Geometry check sheet. Reference: drawing and pictorial views, mm from the part's lowest x, y, z. A direction names the side the tool comes from. Round coordinates to 2 decimals unless told otherwise and drop trailing zeros. Order: outer loops, then holes, each group sorted by start corner. A loop starts at its lowest first (then second) coordinate and runs counter-clockwise, first axis right, second up.
(1) Sectioned sample at C-C (y = 17.3). Record the boundary of the cut face in (x, z), plus the area to 3 significant figures.
(2) Set-up check for the marked faces 4, 5, 6, 7 and 8: record each of +Z, -Z, +X, -X, +Y, -Y from which the full face is reachable in a straight line by a thin tool's end or side.
(3) Release check for a two-part mould opening along X. For the marked faces 1, 2 and 3 record: +X half, -X half, draft (parallel to the pull), parting line (faces both ways), or undercut.
(4) Material ranges on line 1 along Y through (x, z) = (14, 2.6); line 2 along Z through (x, y) = (27, 17.3); line 3 along Y through (x, z) = (13, 1), recorded low to high.
(5) Sectioned sample at B-B (z = 11.5). Record the boundary of the cut face in (x, y), plus the area to 3 significant figures.
(6) Go/stop test with flat-tipped pins: pin 1 (5 mm diameter, centred on x = 16.5, y = 31.5, fed in from +Z); pin 2 (4.5 mm diameter, centred on x = 32, y = 29.5, fed in from -Z); pin 3 (0.6 mm diameter, centred on x = 28.5, y = 34.5, fed in from +Z); pin 4 (3 mm diameter, centred on x = 14, y = 5.3, fed in from +Z). Record where each tip stops, or that it passes through.
(7) Sectioned sample at D-D (z = 2). Record the boundary of the cut face in (x, y).
(8) Sectioned sample at A-A (x = 31). Record the boundary of the cut face in (y, z), plus the area to 3 significant figures.
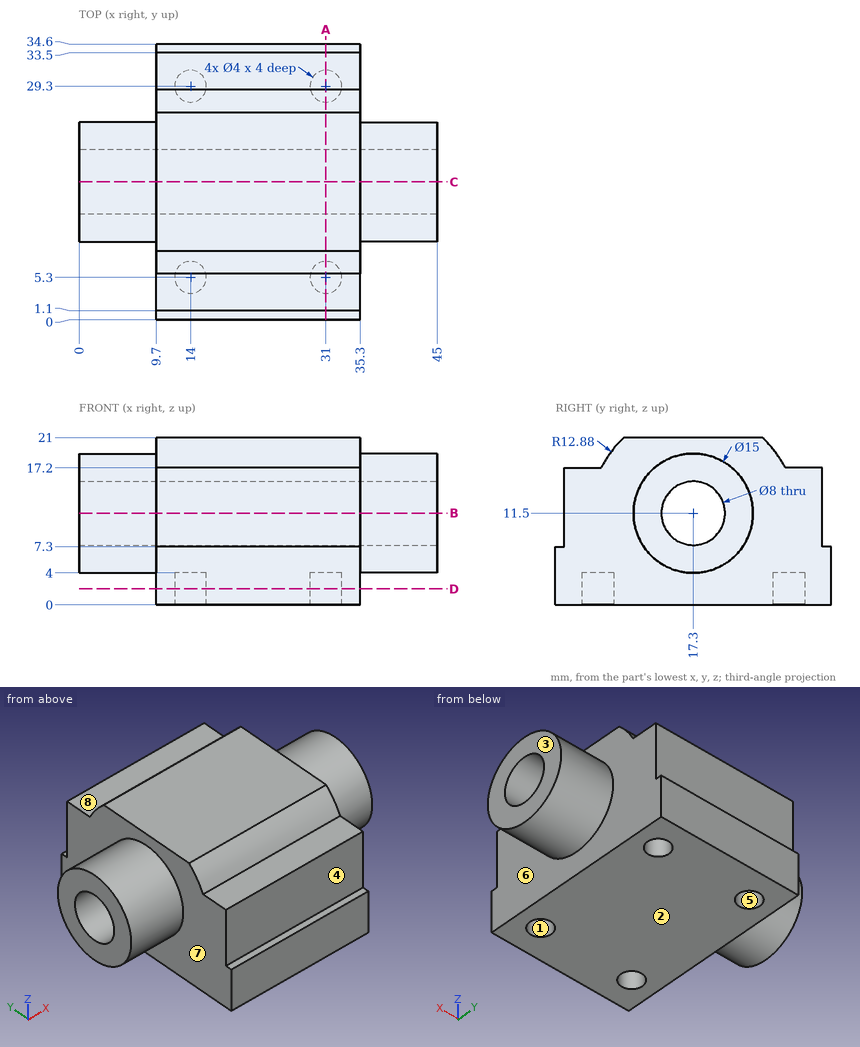
Answer below:
1. outline: (0, 4) - (9.7, 4) - (9.7, 0) - (35.3, 0) - (35.3, 4) - (45, 4) - (45, 7.5) - (0, 7.5) - close; (0, 15.5) - (45, 15.5) - (45, 19) - (35.3, 19) - (35.3, 21) - (9.7, 21) - (9.7, 19) - (0, 19) - close
1. area: 469 mm2
2. face 4: +Z, +X, -X, -Y
2. face 5: -Z
2. face 6: +X
2. face 7: -X
2. face 8: +Z, +X, -X, +Y
3. face 1: undercut
3. face 2: draft
3. face 3: +X half
4. line 1: y = 0 to 3.3, 7.3 to 27.3, 31.3 to 34.6
4. line 2: z = 0 to 7.5, 15.5 to 21
4. line 3: y = 0 to 3.57, 7.03 to 27.57, 31.03 to 34.6
5. outline: (0, 9.8) - (9.7, 9.8) - (9.7, 1.1) - (35.3, 1.1) - (35.3, 9.8) - (45, 9.8) - (45, 13.3) - (0, 13.3) - close; (0, 21.3) - (45, 21.3) - (45, 24.8) - (35.3, 24.8) - (35.3, 33.5) - (9.7, 33.5) - (9.7, 24.8) - (0, 24.8) - close
5. area: 760 mm2
6. pin 1: stops at z = 17.2
6. pin 2: stops at z = 0
6. pin 3: stops at z = 7.3
6. pin 4: stops at z = 18.96
7. outline: (9.7, 0) - (35.3, 0) - (35.3, 34.6) - (9.7, 34.6) - close; hole circle Ø4 at (14, 5.3); hole circle Ø4 at (14, 29.3); hole circle Ø4 at (31, 5.3); hole circle Ø4 at (31, 29.3)
8. outline: (0, 0) - (3.3, 0) - (3.3, 4) - (7.3, 4) - (7.3, 0) - (27.3, 0) - (27.3, 4) - (31.3, 4) - (31.3, 0) - (34.6, 0) - (34.6, 7.3) - (33.5, 7.3) - (33.5, 17.2) - (28.85, 17.2) arc R12.88 ccw to (26, 21) - (8.6, 21) arc R12.88 ccw to (5.75, 17.2) - (1.1, 17.2) - (1.1, 7.3) - (0, 7.3) - close; hole circle Ø8 at (17.3, 11.5)
8. area: 569 mm2
